```python
from build123d import *

# Parameters (mm, degrees)
SKETCH_1_W          = 26.8
SKETCH_1_H          = 28
SKETCH_1_W_2        = 20.8
SKETCH_1_H_2        = 22
EXTRUDE_1_DEPTH     = 30
SKETCH_2_W          = 3
SKETCH_2_H          = 5
CUT_EXTRUDE_1_DEPTH = 30
SKETCH_3_W          = 20.8
SKETCH_3_H          = 1.2
EXTRUDE_2_DEPTH     = 30
SKETCH_4_W          = 26.962863122
SKETCH_4_H          = 1.5
CUT_EXTRUDE_2_DEPTH = 30
SKETCH_5_W          = 7
SKETCH_5_H          = 9
SKETCH_5_W_2        = 3
SKETCH_5_H_2        = 5
CUT_EXTRUDE_3_DEPTH = 47.588517899
EXTRUDE_3_DEPTH     = 5
EXTRUDE_4_DEPTH     = 2.7


with BuildPart() as part:
    # 草图1 → 凸台-拉伸1 (new body)
    with BuildSketch(Plane(origin=(0, 0, 0), x_dir=(0, 0, -1), z_dir=(1, 0, 0))):
        with Locations((10.4, 11)):
            Rectangle(SKETCH_1_W, SKETCH_1_H)
        with Locations((10.4, 11)):
            Rectangle(SKETCH_1_W_2, SKETCH_1_H_2, mode=Mode.SUBTRACT)
    extrude(amount=EXTRUDE_1_DEPTH)

    # 草图2 → 切除-拉伸1 (cut)
    with BuildSketch(Plane(origin=(0, 0, -23.8), x_dir=(-1, 0, 0), z_dir=(0, 0, -1))):
        with Locations((-22.5, 11)):
            Rectangle(SKETCH_2_W, SKETCH_2_H)
        with Locations((-7.5, 11)):
            Rectangle(SKETCH_2_W, SKETCH_2_H)
    extrude(amount=-CUT_EXTRUDE_1_DEPTH, mode=Mode.SUBTRACT)

    # 草图3 → 凸台-拉伸2 (add)
    with BuildSketch(Plane.ZY):
        with Locations((-10.4, 21.4)):
            Rectangle(SKETCH_3_W, SKETCH_3_H)
    extrude(amount=-EXTRUDE_2_DEPTH)

    # 草图4 → 切除-拉伸2 (cut)
    with BuildSketch(Plane.ZY):
        with Locations((-10.318568439, 24.25)):
            Rectangle(SKETCH_4_W, SKETCH_4_H)
    extrude(amount=-CUT_EXTRUDE_2_DEPTH, mode=Mode.SUBTRACT)

    # 草图5 → 切除-拉伸3 (cut, through all)
    # profile 1 of 2: a face of its own
    with BuildSketch(Plane(origin=(0, 0, -23.8), x_dir=(-1, 0, 0), z_dir=(0, 0, -1))):
        with Locations((-22.5, 11)):
            Rectangle(SKETCH_5_W, SKETCH_5_H)
        with Locations((-22.5, 11)):
            Rectangle(SKETCH_5_W_2, SKETCH_5_H_2, mode=Mode.SUBTRACT)
    # profile 2 of 2: a face of its own
    with BuildSketch(Plane(origin=(0, 0, -23.8), x_dir=(-1, 0, 0), z_dir=(0, 0, -1))):
        with Locations((-7.5, 11)):
            Rectangle(SKETCH_5_W, SKETCH_5_H)
        with Locations((-7.5, 11)):
            Rectangle(SKETCH_5_W_2, SKETCH_5_H_2, mode=Mode.SUBTRACT)
    extrude(amount=-CUT_EXTRUDE_3_DEPTH, mode=Mode.SUBTRACT)

    # 草图6 → 凸台-拉伸3 (add)
    with BuildSketch(Plane.XY.offset(3)):
        Polygon((45, 20.8), (45, 46.5), (35.25, 46.5), (35.25, 23.5), (-5.25, 23.5), (-5.25, 46.5), (-15, 46.5), (-15, 20.8), align=None)
        with BuildLine():
            Line((-7.8, 41.8), (-7.8, 26.8))
            ThreePointArc((-7.8, 26.8), (-9.25, 25.35), (-10.7, 26.8))
            Line((-10.7, 26.8), (-10.7, 41.8))
            ThreePointArc((-10.7, 41.8), (-9.25, 43.25), (-7.8, 41.8))
        make_face(mode=Mode.SUBTRACT)
        with BuildLine():
            Line((37.8, 41.8), (37.8, 26.8))
            ThreePointArc((37.8, 26.8), (39.25, 25.35), (40.7, 26.8))
            Line((40.7, 26.8), (40.7, 41.8))
            ThreePointArc((40.7, 41.8), (39.25, 43.25), (37.8, 41.8))
        make_face(mode=Mode.SUBTRACT)
    extrude(amount=-EXTRUDE_3_DEPTH)

    # 草图7 → 凸台-拉伸4 (add)
    with BuildSketch(Plane(origin=(0, 23.5, 0), x_dir=(1, 0, 0), z_dir=(0, 1, 0))):
        Polygon((-10.125, 2), (-10.125, 12.9), (15, 23.8), (40.125, 12.9), (40.125, 2), align=None)
    extrude(amount=-EXTRUDE_4_DEPTH)


solid = part.part
```
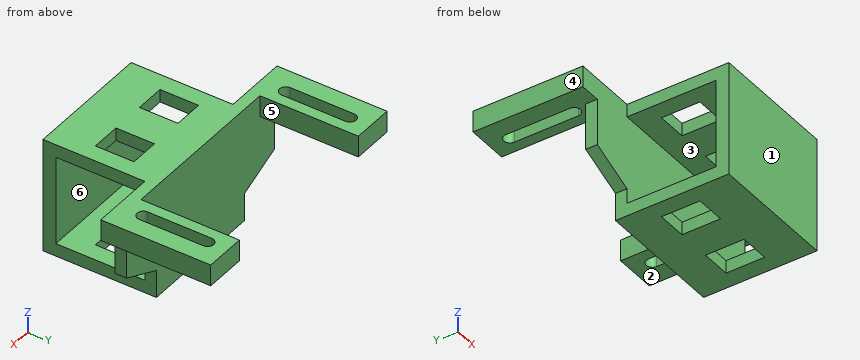
Model file for the job. Use its own axes, mm. Face numbers are marked on the shaded views. A direction names the side the tool comes from. Give positions to 0.01 mm unless a question says otherwise; leave off trailing zeros. Order: outer loops, then holes, each group sorted by start corner. A loop starts at its lowest first (then second) coordinate and runs counter-clockwise, first axis right, second up.
1) Wall check: probe 1 along Y at (x, z) = (22.5, -15); probe 2 along Z at (x, y) = (17, 18.5); probe 3 along Y at (x, z) = (39.5, -10). Give the ranges that are in metal, low to high.
2) Mould opens along Y. For the marked faces 1, 2 and 3 say: +Y half, -Y half, draft (parallel to the pull), parting line (faces both ways), or undercut.
3) Saw through at D-D, the plane x = -9. Write the cut outline in (y, z).
4) 3-axis set-ups, long thin cutter, end or side, ignore diameter. For the marked faces 4, 5 and 6: which of +Z, -Z, +X, -X, +Y, -Y reach the whole face in a straight line?
5) Saw through at B-B, the plane x = 27. Write the cut outline in (y, z).
6) Saw through at C-C, the plane y = 9. Write the cut outline in (x, z), then the cut area to 3 significant figures.
7) Saw through at A-A, the plane z = -19. Write the cut outline in (x, y), then the cut area to 3 significant figures.
8) Pin check, flat tips, straight feed: pin 1 (0.9 mm diameter, centred on y = 9, z = 1.5, fed in from -X); pin 2 (8 mm diameter, centred on x = 15.5, z = -14.5, fed in from +Y); pin 3 (3.5 mm diameter, centred on y = 13, z = 1.5, fed in from +X). Stop position of each tip, or through.
Computed:
1. probe 1: y = -3 to 0, 20.8 to 23.5
1. probe 2: z = -23.8 to -20.8, 0 to 3
1. probe 3: y = 20.8 to 23.5
2. face 1: -Y half
2. face 2: draft
2. face 3: undercut
3. outline: (20.8, -13.39) - (23.5, -13.39) - (23.5, -2) - (25.37, -2) - (25.37, 3) - (20.8, 3) - close; (43.23, -2) - (46.5, -2) - (46.5, 3) - (43.23, 3) - close
4. face 4: +Z, -Z, -X, +Y, -Y
4. face 5: +Z, -Z, +Y
4. face 6: +X, -X
5. outline: (-3, -23.8) - (23.5, -23.8) - (23.5, 3) - (-3, 3) - close; hole (0, -20.8) - (20.8, -20.8) - (20.8, 0) - (0, 0) - close
6. outline: (0, -23.8) - (4, -23.8) - (4, -20.8) - (0, -20.8) - close; (0, 0) - (4, 0) - (4, 3) - (0, 3) - close; (11, -23.8) - (19, -23.8) - (19, -20.8) - (11, -20.8) - close; (11, 0) - (19, 0) - (19, 3) - (11, 3) - close; (26, -23.8) - (30, -23.8) - (30, -20.8) - (26, -20.8) - close; (26, 0) - (30, 0) - (30, 3) - (26, 3) - close
6. area: 96.0 mm2
7. outline: (0, -3) - (30, -3) - (30, 0) - (0, 0) - close; (0, 20.8) - (30, 20.8) - (30, 23.5) - (0, 23.5) - close
7. area: 171 mm2
8. pin 1: stops at x = 0
8. pin 2: stops at y = 23.5
8. pin 3: stops at x = 30
